from build123d import *

# Parameters (mm, degrees)
SKETCH1_W           = 111.125
SKETCH1_H           = 88.9
BOSS_EXTRUDE1_DEPTH = 25.4
SKETCH2_W           = 34.925
SKETCH2_H           = 6.35
CUT_EXTRUDE1_DEPTH  = 108.868259494
SKETCH3_R           = 4.13258
CUT_EXTRUDE2_DEPTH  = 74.266177821


with BuildPart() as part:
    # Sketch1 → Boss-Extrude1 (new body)
    with BuildSketch(Plane(origin=(0, 0, 0), x_dir=(1, 0, 0), z_dir=(0, 1, 0))):
        Rectangle(SKETCH1_W, SKETCH1_H)
    extrude(amount=BOSS_EXTRUDE1_DEPTH)

    # Sketch2 → Cut-Extrude1 (cut, through all)
    with BuildSketch(Plane.XY.offset(44.45)):
        Polygon((-42.8625, 0), (-42.8625, 6.35), (-33.3375, 6.35), (-31.75, 7.9375), (22.225, 7.9375), (23.8125, 6.35), (42.8625, 6.35), (42.8625, 0), align=None)
        with Locations((38.1, 22.225)):
            Rectangle(SKETCH2_W, SKETCH2_H)
    extrude(amount=-CUT_EXTRUDE1_DEPTH, mode=Mode.SUBTRACT)

    # Sketch3 → Cut-Extrude2 (cut, through all)
    with BuildSketch(Plane.XZ.offset(-7.9375)):
        with Locations(Location((-20.962711313, 0.34070329, 0), (0, 0, 270))):
            Circle(SKETCH3_R)
    extrude(amount=-CUT_EXTRUDE2_DEPTH, mode=Mode.SUBTRACT)


solid = part.part
The listing builds one solid part. Answer for the finished solid, in the listing's coordinates (mm). A direction names the side the tool comes from. Coordinates: 2 decimals unless noted, no trailing zeros. Loops run counter-clockwise (first coordinate to the right, second up) from the corner with the lowest first, then second, coordinate; pieces in that order, holes last. Notation, with made-up numbers: (72, 69) -> (121, 69) arc R20 cw to (121, 94) -> close; hole circle Ø7 at (56.25, 65.5). An arc over 180 degrees is marked (long way). Write item = value, one per line. Start each with the question number.
1) A tool of negligible diameter and unlimited length cuts with its end or side. For faces 4 (the face through (38, 19.05, 1)), 5 (the face through (33, 6.35, 1)), 6 (the face through (-10, 25.4, -1)), from which of +Z, -Z, +X, -X, +Y, -Y can it reach the whole face along a straight path? Write none if from no direction.
2) Straight lines are drawn through the part: line 1 (X direction, y = 1.5, z = -12); line 2 (Y direction, x = -25.5, z = -28.5); line 3 (Y direction, x = 40, z = -10). For each, find the intervals that lie inside material, in ascending order. Write a range as from..to.
3) A cutting plane is placed at A-A (y = 3.5). Give the vertices of the cut face in (x, z), then the cut area to 3 significant figures.
4) A cutting plane is placed at D-D (y = 23.25). Give the vertices of the cut face in (x, z).
5) A cutting plane is placed at C-C (x = 1.5). Give the vertices of the cut face in (y, z).
6) Given pin 1 Ø1 at (x, z) = (-36, 28.5) entering from -Y; pin 2 Ø7 at (y, z) = (22, 2) entering from +X; pin 3 Ø12 at (x, z) = (-7.5, 15.5) entering from -Y; pin 4 Ø17.5 at (x, z) = (32.5, -1.5) entering from +Y, each flat-ended and moving along its own axis, determine where each tip first touches the part or whether it passes through.
7) The mould has two halves that part along Z. Classify faces 1 (the face through (49, 0, -1)), 2 (the face through (-1, 15, -44.45)), 3 (the face through (-24.997, 16.547, 1.237)): released by +Z, released by -Z, zero draft, split by the parting line, or undercut.
Responses:
q1.face_4 = +Z, -Z, +X, +Y
q1.face_5 = +Z, -Z, -Y
q1.face_6 = +Z, -Z, +X, -X, +Y
q2.line_1 = -55.56..-42.86, 42.86..55.56
q2.line_2 = 7.94..25.4
q2.line_3 = 6.35..19.05
q3.outline = (-55.56, -44.45) -> (-42.86, -44.45) -> (-42.86, 44.45) -> (-55.56, 44.45) -> close; (42.86, -44.45) -> (55.56, -44.45) -> (55.56, 44.45) -> (42.86, 44.45) -> close
q3.area = 2,260 mm²
q4.outline = (-55.56, -44.45) -> (20.64, -44.45) -> (20.64, 44.45) -> (-55.56, 44.45) -> close; hole circle Ø8.27 at (-20.96, 0.34)
q5.outline = (7.94, -44.45) -> (25.4, -44.45) -> (25.4, 44.45) -> (7.94, 44.45) -> close
q6.pin_1 = 6.35
q6.pin_2 = 55.56
q6.pin_3 = 7.94
q6.pin_4 = 19.05
q7.face_1 = zero draft
q7.face_2 = released by -Z
q7.face_3 = undercut
